```python
from build123d import *

# Parameters (mm, degrees)
F0_R     = 10.9982
F0_R_2   = 11
F1_DEPTH = 7.112


# Not quite as in the source:
# - a feature names something its author has since deleted; it is built from what else it names


with BuildPart() as f1:
    # F0 (on Front) → F1 (new body)
    with BuildSketch(Plane.XZ):
        with BuildLine():
            ThreePointArc((44.45, 0), (40.7302561211, 8.9802561211), (31.75, 12.7))
            ThreePointArc((31.75, 12.7), (19.05, 0), (31.75, -12.7))
            ThreePointArc((31.75, -12.7), (40.7302561211, -8.9802561211), (44.45, 0))
        make_face()
        with Locations((31.75, 0)):
            Circle(F0_R, mode=Mode.SUBTRACT)
        with BuildLine():
            ThreePointArc((-31.75, -12.7), (-22.7697438789, -8.9802561211), (-19.05, 0))
            ThreePointArc((-19.05, 0), (-22.7697438789, 8.9802561211), (-31.75, 12.7))
            ThreePointArc((-31.75, 12.7), (-44.45, 0), (-31.75, -12.7))
        make_face()
        with Locations((-31.75, 0)):
            Circle(F0_R, mode=Mode.SUBTRACT)
        with BuildLine():
            ThreePointArc((-31.75, 12.7), (-22.7697438789, 8.9802561211), (-19.05, 0))
            ThreePointArc((-19.05, 0), (-22.7697438789, -8.9802561211), (-31.75, -12.7))
            Line((-31.75, -12.7), (31.75, -12.7))
            ThreePointArc((31.75, -12.7), (19.05, 0), (31.75, 12.7))
            Line((31.75, 12.7), (-31.75, 12.7))
        make_face()
        Circle(F0_R_2, mode=Mode.SUBTRACT)
    extrude(amount=F1_DEPTH)


solid = f1.part
```
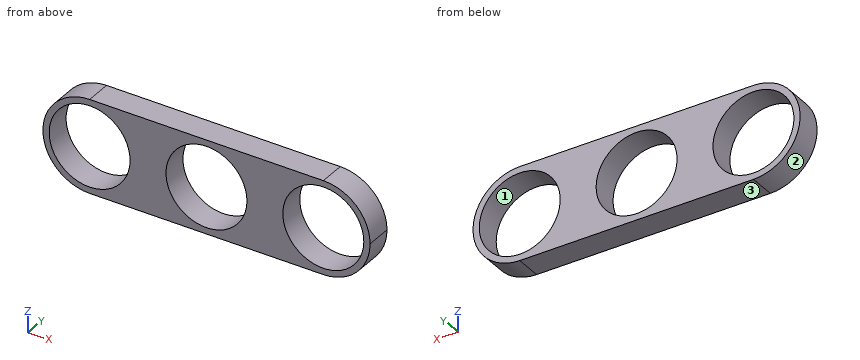
Geometry check sheet. Reference: the model listing, model coordinates, mm. Face numbers are marked on the shaded views. Round coordinates to 2 decimals unless told otherwise and drop trailing zeros. Order: outer loops, then holes, each group sorted by start corner. A loop starts at its lowest first (then second) coordinate and runs counter-clockwise, first axis right, second up. Notation, with made-up numbers: (71.25, 20) - (122.25, 20) arc R16 ccw to (122.25, 26) - close; hole circle Ø10 at (83, 75). An arc over 180 degrees is marked (long way). Use a Markdown table: item, result. Add a question column.
(1) Material ranges on line 1 along Z through (x, y) = (-31.75, -4); line 2 along X through (y, z) = (-4.5, 6.5); line 3 along X through (y, z) = (-6.25, -3.75), recorded low to high. Write a range as [from, to].
(2) Sectioned sample at C-C, the plane y = -3. Enter the section's corners in (x, z).
(3) Depth check by flat-ended pin: pin 1 (1.5 mm diameter, centred on x = 35.5, y = -5.5, fed in from -Z); pin 2 (1 mm diameter, centred on x = -6, z = -6.5, fed in from +Y). Enter the tip coordinate at first touch or a pass-through.
(4) Release check for a two-part mould opening along X. For the marked faces 1, 2 and 3 record: pulls with the +X half, pulls with the -X half, needs draft (parallel to the pull), parting line crosses it, or undercut.
(5) Sectioned sample at A-A, the plane x = 0. Enter the section's corners in (y, z).
(6) Sectioned sample at D-D, the plane x = 21.5. Enter the section's corners in (y, z), and give its area (3 significant figures).
(7) Sectioned sample at B-B, the plane z = 9. Enter the section's corners in (x, y), and give its area (3 significant figures).
Answers below:
| question | item | result |
|---|---|---|
| 1 | line 1 | [-12.7, -11], [11, 12.7] |
| 1 | line 2 | [-42.66, -40.62], [-22.88, -8.87], [8.87, 22.88], [40.62, 42.66] |
| 1 | line 3 | [-43.88, -42.09], [-21.41, -10.34], [10.34, 21.41], [42.09, 43.88] |
| 2 | outline | (-31.75, -12.7) - (31.75, -12.7) arc R12.7 ccw to (31.75, 12.7) - (-31.75, 12.7) arc R12.7 ccw to start; hole circle Ø22 at (-31.75, 0); hole circle Ø22 at (0, 0); hole circle Ø22 at (31.75, 0) |
| 3 | pin 1 | z = -12.34 |
| 3 | pin 2 | through |
| 4 | face 1 | undercut |
| 4 | face 2 | pulls with the -X half |
| 4 | face 3 | needs draft |
| 5 | outline | (-7.11, -12.7) - (0, -12.7) - (0, -11) - (-7.11, -11) - close; (-7.11, 11) - (0, 11) - (0, 12.7) - (-7.11, 12.7) - close |
| 6 | outline | (-7.11, -12.7) - (0, -12.7) - (0, -3.99) - (-7.11, -3.99) - close; (-7.11, 3.99) - (0, 3.99) - (0, 12.7) - (-7.11, 12.7) - close |
| 6 | area | 124 mm² |
| 7 | outline | (-40.71, -7.11) - (-38.07, -7.11) - (-38.07, 0) - (-40.71, 0) - close; (-25.43, -7.11) - (-6.32, -7.11) - (-6.32, 0) - (-25.43, 0) - close; (6.32, -7.11) - (25.43, -7.11) - (25.43, 0) - (6.32, 0) - close; (38.07, -7.11) - (40.71, -7.11) - (40.71, 0) - (38.07, 0) - close |
| 7 | area | 309 mm² |
